from build123d import *

# Parameters (mm, degrees)
SKETCH1_W           = 337
SKETCH1_H           = 181
BOSS_EXTRUDE1_DEPTH = 25.4
SHELL1_T            = -5
SKETCH2_W           = 286.2
SKETCH2_H           = 130.2
CUT_EXTRUDE1_DEPTH  = 193.944707105


with BuildPart() as part:
    # Sketch1 → Boss-Extrude1 (new body)
    with BuildSketch(Plane(origin=(0, 0, 0), x_dir=(1, 0, 0), z_dir=(0, 1, 0))):
        Rectangle(SKETCH1_W, SKETCH1_H)
    extrude(amount=BOSS_EXTRUDE1_DEPTH)

    # Shell1
    shell1_openings = [part.faces().sort_by_distance(p)[0] for p in [
        (0, 25.4, 0),
    ]]
    offset(amount=SHELL1_T, openings=shell1_openings, kind=Kind.INTERSECTION)

    # Sketch2 → Cut-Extrude1 (cut, through all)
    with BuildSketch(Plane.XZ):
        Rectangle(SKETCH2_W, SKETCH2_H)
    extrude(amount=-CUT_EXTRUDE1_DEPTH, mode=Mode.SUBTRACT)


solid = part.part
Can you work these out from the model? Positions are in its coordinate system, mm. A direction names the side the tool comes from. Give positions to 0.01 mm unless a question says otherwise; leave off trailing zeros. Order: outer loops, then holes, each group sorted by start corner. A loop starts at its lowest first (then second) coordinate and runs counter-clockwise, first axis right, second up. Notation, with made-up numbers: M 73.5,62.5 L 125.5,62.5 A14 ccw 125.5,82.5 Z; hole C 87,51 d10. An arc over 180 degrees is marked long. Use one line per item in the form item = value. Start each with the question number.
Item 1: For faces 1 (the flat face through (-1, 25.4, -88)), 2 (the flat face through (163.5, 15, 1)), which set-ups out of +Z, -Z, +X, -X, +Y, -Y let a thin tool reach every point of the face, with its end or its side?
Item 2: If I drill on line 1 along Z through (x, y) = (-29, 3.5); line 2 along X through (y, z) = (5.5, -59.5); line 3 along Z through (x, y) = (65.5, 8.5), over which ranges is the centre line in solid material (lowest first)?
Item 3: If we section it at C-C (z = -55): Write out the boundary of the cut face in (x, y), then the cut area to 3 significant figures.
Item 4: If we section it at A-A (x = 28): Write out the boundary of the cut face in (y, z), then the cut area to 3 significant figures.
Item 5: If we section it at B-B (y = 19.25): Write out the boundary of the cut face in (x, z).
Item 6: We'd pull the mould along Z, two halves only. Please class faces 3 (the flat face through (-2, 13, 90.5)), 4 (the flat face through (-2, 13, -90.5)), 5 (the flat face through (-2, 15, 85.5)), 6 (the flat face through (-168.5, 13, 1)): +Z half, -Z half, draft (parallel to the pull), parting line (faces both ways), or undercut.
Outcome:
q1.face_1 = +Z, -Z, +X, -X, +Y
q1.face_2 = +Y
q2.line_1 = -90.5 to -65.1, 65.1 to 90.5
q2.line_2 = -168.5 to -163.5, 163.5 to 168.5
q2.line_3 = -90.5 to -85.5, 85.5 to 90.5
q3.outline = M -168.5,0 L -143.1,0 L -143.1,5 L -163.5,5 L -163.5,25.4 L -168.5,25.4 Z; M 143.1,0 L 168.5,0 L 168.5,25.4 L 163.5,25.4 L 163.5,5 L 143.1,5 Z
q3.area = 458 mm2
q4.outline = M 0,-90.5 L 25.4,-90.5 L 25.4,-85.5 L 5,-85.5 L 5,-65.1 L 0,-65.1 Z; M 0,65.1 L 5,65.1 L 5,85.5 L 25.4,85.5 L 25.4,90.5 L 0,90.5 Z
q4.area = 458 mm2
q5.outline = M -168.5,-90.5 L 168.5,-90.5 L 168.5,90.5 L -168.5,90.5 Z; hole M -163.5,-85.5 L 163.5,-85.5 L 163.5,85.5 L -163.5,85.5 Z
q6.face_3 = +Z half
q6.face_4 = -Z half
q6.face_5 = undercut
q6.face_6 = draft
